from build123d import *

# Parameters (mm, degrees)
SKETCH_1_R      = 11.05
SKETCH_1_R_2    = 2.75
SKETCH_1_R_3    = 1.25
SKETCH_1_R_4    = 4.25
EXTRUDE_1_DEPTH = 3


with BuildPart() as part:
    # 草图1 → 凸台-拉伸1 (new body)
    with BuildSketch(Plane.XY):
        with BuildLine():
            Line((-40, 20), (-40, -37))
            ThreePointArc((-40, -37), (-38.535533906, -40.535533906), (-35, -42))
            Line((-35, -42), (35, -42))
            ThreePointArc((35, -42), (38.535533906, -40.535533906), (40, -37))
            Line((40, -37), (40, 20))
            ThreePointArc((40, 20), (38.535533906, 23.535533906), (35, 25))
            Line((35, 25), (-35, 25))
            ThreePointArc((-35, 25), (-38.535533906, 23.535533906), (-40, 20))
        make_face()
        Circle(SKETCH_1_R, mode=Mode.SUBTRACT)
        with Locations((-25, 16)):
            Circle(SKETCH_1_R_2, mode=Mode.SUBTRACT)
        with Locations((-25, -16)):
            Circle(SKETCH_1_R_2, mode=Mode.SUBTRACT)
        with Locations((25, -16)):
            Circle(SKETCH_1_R_2, mode=Mode.SUBTRACT)
        with Locations((25, 16)):
            Circle(SKETCH_1_R_2, mode=Mode.SUBTRACT)
        with Locations((0, -32)):
            Circle(SKETCH_1_R_3, mode=Mode.SUBTRACT)
        with Locations((-20, -32)):
            Circle(SKETCH_1_R_3, mode=Mode.SUBTRACT)
        with Locations((20, -32)):
            Circle(SKETCH_1_R_3, mode=Mode.SUBTRACT)
        with Locations((-25, 0)):
            Circle(SKETCH_1_R_4, mode=Mode.SUBTRACT)
        with Locations((25, 0)):
            Circle(SKETCH_1_R_4, mode=Mode.SUBTRACT)
        with Locations((0, 18)):
            Circle(SKETCH_1_R_2, mode=Mode.SUBTRACT)
        with Locations((0, -18)):
            Circle(SKETCH_1_R_2, mode=Mode.SUBTRACT)
    extrude(amount=EXTRUDE_1_DEPTH)


solid = part.part
The model under review builds one solid part; all positions refer to its coordinate system, in mm. Coordinates: 2 decimals unless noted, no trailing zeros. Loops run counter-clockwise (first coordinate to the right, second up) from the corner with the lowest first, then second, coordinate; pieces in that order, holes last. Notation, with made-up numbers: M -13.5,54.5 L 27.5,54.5 A26 ccw 27.5,84.5 Z; hole C -12,6.5 d7. An arc over 180 degrees is marked long. Put each result on its own line as item: value. Start each with the question number.
Q1. Add section C-C (y = 0). Write out the cut boundary in (x, z), and give its area (3 significant figures).
Q2. Add section B-B (z = 0.9). Count the separate pieces of the cut face and the enclosed holes in it, and give its area (3 significant figures).
Q3. Wall thickness on line 1 (Y direction, x = 25, z = 2.05); line 2 (Y direction, x = 0, z = 1.5); line 3 (Y direction, x = -20, z = 1.65): over which ranges is each line inside the solid? List them lowest first.
Q4. Add section A-A (x = 25). Write out the cut boundary in (y, z).
Q5. The part is to be moulded in two halves that separate along X. For faces 1 (the cylindrical face through (-39, -40, 1)), 2 (the cylindrical face through (-28.132, 2.872, 1.479)), 3 (the flat face through (-9, -8, 0)), say which applies: +X half, -X half, draft (parallel to the pull), parting line (faces both ways), or undercut.
Q6. Clearance check with flat-ended pins moving along their axes: pin 1 (7 mm diameter, centred on x = -25, y = 16, fed in from +Z); pin 2 (13.5 mm diameter, centred on x = 0, y = 0, fed in from +Z). State where each tip first meets the part, or that it passes through.
Q7. Add section D-D (x = 0). Write out the cut boundary in (y, z).
Answers:
1. outline: M -40,0 L -29.25,0 L -29.25,3 L -40,3 Z; M -20.75,0 L -11.05,0 L -11.05,3 L -20.75,3 Z; M 11.05,0 L 20.75,0 L 20.75,3 L 11.05,3 Z; M 29.25,0 L 40,0 L 40,3 L 29.25,3 Z
1. area: 123 mm^2
2. separate pieces: 1
2. enclosed holes: 12
2. area: 4,680 mm^2
3. line 1: y = -42 to -18.75, -13.25 to -4.25, 4.25 to 13.25, 18.75 to 25
3. line 2: y = -42 to -33.25, -30.75 to -20.75, -15.25 to -11.05, 11.05 to 15.25, 20.75 to 25
3. line 3: y = -42 to -33.25, -30.75 to 25
4. outline: M -42,0 L -18.75,0 L -18.75,3 L -42,3 Z; M -13.25,0 L -4.25,0 L -4.25,3 L -13.25,3 Z; M 4.25,0 L 13.25,0 L 13.25,3 L 4.25,3 Z; M 18.75,0 L 25,0 L 25,3 L 18.75,3 Z
5. face 1: -X half
5. face 2: undercut
5. face 3: draft
6. pin 1: stops at z = 3
6. pin 2: passes through
7. outline: M -42,0 L -33.25,0 L -33.25,3 L -42,3 Z; M -30.75,0 L -20.75,0 L -20.75,3 L -30.75,3 Z; M -15.25,0 L -11.05,0 L -11.05,3 L -15.25,3 Z; M 11.05,0 L 15.25,0 L 15.25,3 L 11.05,3 Z; M 20.75,0 L 25,0 L 25,3 L 20.75,3 Z
